Input: part model. Units: mm. Frame: model coordinates. A direction names the side the tool comes from. Coordinates: 2 decimals unless noted, no trailing zeros. Order: outer loops, then holes, each group sorted by start corner. A loop starts at its lowest first (then second) coordinate and runs counter-clockwise, first axis right, second up. Notation, with made-up numbers: (-22, 62) -> (10, 62) arc R37 cw to (10, 100) -> close; hole circle Ø9 at (-31.75, -6). An arc over 180 degrees is marked (long way). Use one line per item in the form item = value. Start each with the question number.
1) Section query B-B on x = 4.5. Output: boundary loops of the cut face in (y, z).
2) Draft query along Z for faces 1 (the flat face through (3, -3, 88.9)), 2 (the flat face through (3, 0, -29)), 3 (the flat face through (3, 27, -132.7)), 4 (the flat face through (3, 55, 111)). Return one class per face: pulls with the +Z half, pulls with the -Z half, needs draft (parallel to the pull), parting line crosses it, or undercut.
3) Ray query, line 1 along Z through (x, y) = (3, 86.5); line 2 along Z through (x, y) = (2.5, 10); line 3 along Y through (x, z) = (2.5, -10.5). Return the intervals inside material, ascending.
4) Section query A-A on y = 83. Output: boundary loops of the cut face in (x, z), then the cut area to 3 significant figures.
5) Section query C-C on z = 93.5. Output: boundary loops of the cut face in (x, y).
6) Section query D-D on z = -8. Output: boundary loops of the cut face in (x, y).
7) Access query for faces 5 (the flat face through (3, 0, 29)), 6 (the flat face through (3, 0, -111)), 7 (the flat face through (3, 77, -38.1)), 8 (the flat face through (3, 77, 88.9)). Directions: +Z, -Z, +X, -X, +Y, -Y. A direction counts if a zero-diameter tool reaches every point of the face in a straight line with its end or side. Return the directions, or none.
8) Pin query (flat end, axial travel): pin 1 (1.5 mm diameter, centred on x = 2, z = 30, fed in from -Y); pin 2 (3 mm diameter, centred on x = 3, y = 80.5, fed in from +Z); pin 3 (2 mm diameter, centred on x = 2.5, y = 68.5, fed in from -Z). Return the tip coordinate at first contact, or that it passes through.
from build123d import *

# Parameters (mm, degrees)
BOSS_EXTRUDE1_DEPTH = 6.35
SKETCH4_W           = 6.35
SKETCH4_H           = 237.700000096
SKETCH4_H_2         = 112.7
BOSS_EXTRUDE2_DEPTH = 6.35
SKETCH5_W           = 6.35
SKETCH5_H           = 390.400000096
BOSS_EXTRUDE3_DEPTH = 6.35
SKETCH6_W           = 125.000000096
SKETCH6_H           = 67.700000012
CUT_EXTRUDE1_DEPTH  = 265.978178443
SKETCH7_W           = 76.2
SKETCH7_H           = 6.35
CUT_EXTRUDE2_DEPTH  = 147.333301068
SKETCH8_W           = 6.35
SKETCH8_H           = 50.8
BOSS_EXTRUDE4_DEPTH = 38.1


with BuildPart() as part:
    # Sketch3 → Boss-Extrude1 (new body)
    with BuildSketch(Plane(origin=(0, 0, 0), x_dir=(0, 0, -1), z_dir=(1, 0, 0))):
        Polygon((-132.7, 55.000000012), (-132.7, 0), (-20, 0), (-20, 35), (20, 35), (20, 0), (257.700000096, 0), (257.700000096, 55.000000012), align=None)
    extrude(amount=BOSS_EXTRUDE1_DEPTH)

    # Sketch4 → Boss-Extrude2 (add)
    with BuildSketch(Plane.XZ):
        with Locations((3.175, -138.850000048)):
            Rectangle(SKETCH4_W, SKETCH4_H)
        with Locations((3.175, 76.35)):
            Rectangle(SKETCH4_W, SKETCH4_H_2)
    extrude(amount=BOSS_EXTRUDE2_DEPTH)

    # Sketch5 → Boss-Extrude3 (add)
    with BuildSketch(Plane(origin=(0, 55.000000012, 0), x_dir=(1, 0, 0), z_dir=(0, 1, 0))):
        with Locations((3.175, 62.500000048)):
            Rectangle(SKETCH5_W, SKETCH5_H)
    extrude(amount=BOSS_EXTRUDE3_DEPTH)

    # Sketch6 → Cut-Extrude1 (cut, through all)
    with BuildSketch(Plane(origin=(6.35, 0, 0), x_dir=(0, 0, -1), z_dir=(1, 0, 0))):
        with Locations((195.200000048, 27.500000006)):
            Rectangle(SKETCH6_W, SKETCH6_H)
    extrude(amount=-CUT_EXTRUDE1_DEPTH, mode=Mode.SUBTRACT)

    # Sketch7 → Cut-Extrude2 (cut, through all)
    with BuildSketch(Plane(origin=(6.35, 0, 0), x_dir=(0, 0, -1), z_dir=(1, 0, 0))):
        Polygon((-88.9, 0), (-126.35, 0), (-132.7, 0), (-132.7, -6.35), (-88.9, -6.35), align=None)
        Polygon((-26.35, 0), (-38.1, 0), (-38.1, -6.35), (-20, -6.35), (-20, 0), align=None)
        Polygon((26.35, 0), (20, 0), (20, -6.35), (38.1, -6.35), (38.1, 0), align=None)
        Polygon((132.7, 0), (126.35, 0), (88.9, 0), (88.9, -6.35), (132.7, -6.35), align=None)
        Polygon((88.9, 61.350000012), (88.9, 55.000000012), (126.35, 55.000000012), (132.7, 55.000000012), (132.7, 61.350000012), align=None)
        with Locations((0, 58.175000012)):
            Rectangle(SKETCH7_W, SKETCH7_H)
        Polygon((-132.7, 55.000000012), (-126.35, 55.000000012), (-88.9, 55.000000012), (-88.9, 61.350000012), (-132.7, 61.350000012), align=None)
    extrude(amount=-CUT_EXTRUDE2_DEPTH, mode=Mode.SUBTRACT)

    # Sketch8 → Boss-Extrude4 (add)
    with BuildSketch(Plane(origin=(0, 61.350000012, 0), x_dir=(1, 0, 0), z_dir=(0, 1, 0))):
        with Locations((3.175, 63.5)):
            Rectangle(SKETCH8_W, SKETCH8_H)
        with Locations((3.175, -63.5)):
            Rectangle(SKETCH8_W, SKETCH8_H)
    extrude(amount=BOSS_EXTRUDE4_DEPTH)


solid = part.part
Answers below:
q1.outline = (-6.35, -88.9) -> (0, -88.9) -> (0, -132.7) -> (55, -132.7) -> (55, -88.9) -> (99.45, -88.9) -> (99.45, -38.1) -> (55, -38.1) -> (55, 38.1) -> (99.45, 38.1) -> (99.45, 88.9) -> (55, 88.9) -> (55, 132.7) -> (0, 132.7) -> (0, 88.9) -> (-6.35, 88.9) -> (-6.35, 38.1) -> (0, 38.1) -> (0, 20) -> (35, 20) -> (35, -20) -> (0, -20) -> (0, -38.1) -> (-6.35, -38.1) -> close
q2.face_1 = pulls with the +Z half
q2.face_2 = undercut
q2.face_3 = pulls with the -Z half
q2.face_4 = needs draft
q3.line_1 = -88.9 to -38.1, 38.1 to 88.9
q3.line_2 = -132.7 to -20, 20 to 132.7
q3.line_3 = 35 to 55
q4.outline = (0, -88.9) -> (6.35, -88.9) -> (6.35, -38.1) -> (0, -38.1) -> close; (0, 38.1) -> (6.35, 38.1) -> (6.35, 88.9) -> (0, 88.9) -> close
q4.area = 645 mm^2
q5.outline = (0, 0) -> (6.35, 0) -> (6.35, 55) -> (0, 55) -> close
q6.outline = (0, 35) -> (6.35, 35) -> (6.35, 55) -> (0, 55) -> close
q7.face_5 = +X, -X, -Y
q7.face_6 = -Z, +X, -X, -Y
q7.face_7 = +X, -X, +Y
q7.face_8 = +Z, +X, -X, +Y
q8.pin_1 = 0
q8.pin_2 = 88.9
q8.pin_3 = -88.9
